Geometry check sheet. Reference: the model listing, model coordinates, mm. A direction names the side the tool comes from. Coordinates: 2 decimals unless noted, no trailing zeros. Loops run counter-clockwise (first coordinate to the right, second up) from the corner with the lowest first, then second, coordinate; pieces in that order, holes last. Notation, with made-up numbers: (-40, 52.5) - (8, 52.5) arc R24 ccw to (8, 63.5) - close; hole circle Ø8 at (14.25, -36). An arc over 180 degrees is marked (long way). Write item = value, one per line. Start each with the question number.
from build123d import *

# Parameters (mm, degrees)
F1_R     = 30
F1_R_2   = 25
F3_R     = 82.5
F4_DEPTH = 15


with BuildPart() as f2:
    # F2: sweep along a path in F0
    with BuildLine(Plane.YZ) as f2_path:
        Line((0, 0), (0, -50))
        Line((0, -50), (0, -650))
    # F1 (on Top) → F2 (sweep)
    with BuildSketch(Plane.XY):
        Circle(F1_R)
        Circle(F1_R_2, mode=Mode.SUBTRACT)
    sweep(path=f2_path.line)

    # F3 (on Top) → F4 (join)
    with BuildSketch(Plane.XY):
        Circle(F3_R)
    extrude(amount=-F4_DEPTH)

    # F5 (on Front) → F6 (revolve)
    with BuildSketch(Plane.XZ):
        with BuildLine():
            Line((50, -650), (35, -650))
            Line((35, -650), (30, -650))
            Line((30, -650), (20, -650))
            Line((20, -650), (20, -715))
            Line((20, -715), (30, -715))
            Line((30, -715), (40, -705))
            Line((40, -705), (40, -695))
            ThreePointArc((40, -695), (37.844933, -687.5), (40, -680))
            Line((40, -680), (40, -660))
            Line((40, -660), (50, -660))
            Line((50, -660), (50, -650))
        make_face()
    revolve(axis=Axis((0, 0, 0), (0, 0, -1)))


solid = f2.part
(1) Draft check along Y on faces 4 (the face through (-4.336, 19.524, -682.955)), 5 (the face through (-1, 1, 0)), 6 (the face through (-3.987, -30.365, -714.374)). Enter one of: pulls with the +Y half, pulls with the -Y half, needs draft (parallel to the pull), parting line crosses it, or undercut.
(2) Tool access check on faces 1 (the face through (-17.88, -80.54, -7.4)), 2 (the face through (-11, -17, -650)), 3 (the face through (22, -34, -660)). Record the directions out of +Z, -Z, +X, -X, +Y, -Y that give a thin tool (end or side, any length) a straight path to the whole face; none if there is none.
(3) Scan lines: line 1 (Y direction, x = 0, z = -224); line 2 (Z direction, x = 38.5, y = 20). Record each from-to range of solid material in increasing order.
(4) Sectioned sample at D-D on y = 69. Enter the section's corners in (x, z).
(5) Sectioned sample at C-C on z = -626. Enter the section's corners in (x, y), plus the area to 3 significant figures.
(6) Depth check by flat-ended pin: pin 1 (2 mm diameter, centred on y = -26.5, z = -151, fed in from -X); pin 2 (8 mm diameter, centred on x = 13, z = -553, fed in from +Y); pin 3 (4 mm diameter, centred on x = 33.5, z = -609.5, fed in from -Y); pin 4 (6 mm diameter, centred on y = -3, z = -253, fed in from -X). Enter the tip coordinate at first touch or a pass-through.
Working result:
q1.face_4 = undercut
q1.face_5 = needs draft
q1.face_6 = parting line crosses it
q2.face_1 = +Z, -Z
q2.face_2 = none
q2.face_3 = -Z
q3.line_1 = -30 to -25, 25 to 30
q3.line_2 = -660 to -650, -15 to 0
q4.outline = (-45.22, -15) - (45.22, -15) - (45.22, 0) - (-45.22, 0) - close
q5.outline = circle Ø60 at (0, 0); hole circle Ø50 at (0, 0)
q5.area = 864 mm2
q6.pin_1 = -15.8
q6.pin_2 = 28.62
q6.pin_3 = through
q6.pin_4 = -30
